from build123d import *

# Parameters (mm, degrees)
SKETCH1_W           = 20
SKETCH1_H           = 20
BOSS_EXTRUDE1_DEPTH = 4.15
SKETCH4_R           = 1.125
BOSS_EXTRUDE3_DEPTH = 0.35
SKETCH5_W           = 14.6
SKETCH5_H           = 14.6
BOSS_EXTRUDE4_DEPTH = 0.01
FILLET1_R           = 0.55
CHAMFER1_SIZE       = 0.5
CUT_EXTRUDE1_DEPTH  = 15.73847007
SKETCH7_R           = 0.4
BOSS_EXTRUDE5_DEPTH = 2


with BuildPart() as part:
    # Sketch1 → Boss-Extrude1 (new body)
    with BuildSketch(Plane.XY):
        Rectangle(SKETCH1_W, SKETCH1_H)
    extrude(amount=BOSS_EXTRUDE1_DEPTH)

    # Sketch4 → Boss-Extrude3 (add)
    with BuildSketch(Plane.XY.offset(4.15)):
        with Locations((0, 1.6)):
            Circle(SKETCH4_R)
    extrude(amount=BOSS_EXTRUDE3_DEPTH)

    # Sketch5 → Boss-Extrude4 (add)
    with BuildSketch(Plane.XY.offset(4.15)):
        with Locations((0, 0.7)):
            Rectangle(SKETCH5_W, SKETCH5_H)
    extrude(amount=BOSS_EXTRUDE4_DEPTH)

    # Fillet1
    # the kernel refuses this fillet: 0.55 mm, written as the material it adds along each edge
    with BuildSketch(Plane(origin=(0, 1.6, 4.16), x_dir=(1, 0, 0), z_dir=(0, 1, 0))) as fillet1_piece_1:
        with BuildLine():
            CenterArc((1.633330601, -0.55), FILLET1_R, 90, 67.553649419)
            Line((1.125, -0.34), (1.114833388, -0.3358))
            ThreePointArc((1.114833388, -0.3358), (1.114, -0.17), (1.114, 0))
            Line((1.114, 0), (1.125, 0.011))
            Line((1.125, 0.011), (1.633330601, 0.011))
            Line((1.633330601, 0.011), (1.633330601, 0))
        make_face()
    revolve(axis=Axis((0, 1.6, 4.16), (0, 0, -1)))

    # Chamfer1
    chamfer1_edges = [part.edges().sort_by_distance(p)[0] for p in [
        (-7.3, -6.6, 4.155),
        (7.3, 8, 4.155),
    ]]
    chamfer(chamfer1_edges, length=CHAMFER1_SIZE)

    # Sketch6 → Cut-Extrude1 (cut, through all)
    with BuildSketch(Plane.XY.offset(4.15)):
        Polygon((7.960512242, -10), (10, -7.960512242), (10, -10), align=None)
        with BuildLine():
            Line((10, 7.966904756), (10, 10))
            Line((10, 10), (7.966904756, 10))
            ThreePointArc((7.966904756, 10), (9.40452019, 9.40452019), (10, 7.966904756))
        make_face()
        with BuildLine():
            Line((-7.966904756, 10), (-10, 10))
            Line((-10, 10), (-10, 7.966904756))
            ThreePointArc((-10, 7.966904756), (-9.40452019, 9.40452019), (-7.966904756, 10))
        make_face()
        with BuildLine():
            Line((-10, -7.966904756), (-10, -10))
            Line((-10, -10), (-7.966904756, -10))
            ThreePointArc((-7.966904756, -10), (-9.40452019, -9.40452019), (-10, -7.966904756))
        make_face()
    extrude(amount=-CUT_EXTRUDE1_DEPTH, mode=Mode.SUBTRACT)

    # Sketch7 → Boss-Extrude5 (add)
    with BuildSketch(Plane(origin=(0, 0, 0), x_dir=(-1, 0, 0), z_dir=(0, 0, -1))):
        with Locations(Location((0, 1.6, 0), (0, 0, 180))):
            Circle(SKETCH7_R)
    extrude(amount=BOSS_EXTRUDE5_DEPTH)


solid = part.part
Verification items for the finished model (mm, model axes). Give positions to 0.01 mm unless a question says otherwise; leave off trailing zeros. Loops run counter-clockwise (first coordinate to the right, second up) from the corner with the lowest first, then second, coordinate; pieces in that order, holes last.
1) Depth check by flat-ended pin: pin 1 Ø6 at (x, y) = (2.5, 4.5) entering from -Z. Enter the tip coordinate at first touch or a pass-through.
2) Sectioned sample at B-B, the plane x = 0. Enter the section's corners in (y, z) (3 decimals).
3) Thickness scan on line 1 along Z through (x, y) = (0, 9); line 2 along X through (y, z) = (1.25, -1.5); line 3 along Y through (x, z) = (-8.75, 2.75). Record the ranges inside material, lowest first.
4) Sectioned sample at C-C, the plane y = 1.6. Enter the section's corners in (x, z) (3 decimals), then the cut area to 3 significant figures.
5) Sectioned sample at D-D, the plane z = -0.25. Enter the section's corners in (x, y).
Answers:
1. pin 1: stops at z = 0
2. outline: (-10, 0) - (1.2, 0) - (1.2, -2) - (2, -2) - (2, 0) - (10, 0) - (10, 4.15) - (8, 4.15) - (8, 4.16) - (3.233, 4.16) arc R0.55 cw to (2.725, 4.5) - (0.475, 4.5) arc R0.55 cw to (-0.033, 4.16) - (-6.6, 4.16) - (-6.6, 4.15) - (-10, 4.15) - close
3. line 1: z = 0 to 4.15
3. line 2: x = -0.19 to 0.19
3. line 3: y = -9.84 to 9.84
4. outline: (-10, 0) - (-0.4, 0) - (-0.4, -2) - (0.4, -2) - (0.4, 0) - (10, 0) - (10, 4.15) - (7.3, 4.15) - (7.3, 4.16) - (1.633, 4.16) arc R0.55 cw to (1.125, 4.5) - (-1.125, 4.5) arc R0.55 cw to (-1.633, 4.16) - (-7.3, 4.16) - (-7.3, 4.15) - (-10, 4.15) - close
4. area: 85.6 mm2
5. outline: circle Ø0.8 at (0, 1.6)
